from build123d import *

# Parameters (mm, degrees)
SKETCH_1_R          = 1.5
SKETCH_1_R_2        = 10
EXTRUDE_1_DEPTH     = 0.7
SKETCH_2_R          = 1.5
CUT_EXTRUDE_1_DEPTH = 40
SKETCH_4_R          = 1.5
CUT_EXTRUDE_2_DEPTH = 10


with BuildPart() as part:
    # 草图1 → 凸台-拉伸1 (new body)
    with BuildSketch(Plane.XY):
        with BuildLine():
            Line((20, 100), (-20, 100))
            ThreePointArc((-20, 100), (-76.568542495, 76.568542495), (-100, 20))
            Line((-100, 20), (-100, -80))
            ThreePointArc((-100, -80), (-94.142135624, -94.142135624), (-80, -100))
            Line((-80, -100), (80, -100))
            ThreePointArc((80, -100), (94.142135624, -94.142135624), (100, -80))
            Line((100, -80), (100, 20))
            ThreePointArc((100, 20), (76.568542495, 76.568542495), (20, 100))
        make_face()
        with Locations((-90, -90)):
            Circle(SKETCH_1_R, mode=Mode.SUBTRACT)
        with Locations((-66, -90)):
            Circle(SKETCH_1_R, mode=Mode.SUBTRACT)
        with Locations((-90, -60)):
            Circle(SKETCH_1_R, mode=Mode.SUBTRACT)
        with Locations((-66, -60)):
            Circle(SKETCH_1_R, mode=Mode.SUBTRACT)
        with Locations((-29, -90)):
            Circle(SKETCH_1_R, mode=Mode.SUBTRACT)
        with Locations((-45, -75)):
            Circle(SKETCH_1_R_2, mode=Mode.SUBTRACT)
        with Locations((-50, -36)):
            Circle(SKETCH_1_R, mode=Mode.SUBTRACT)
        with Locations((-50, -27)):
            Circle(SKETCH_1_R, mode=Mode.SUBTRACT)
        with BuildLine():
            ThreePointArc((-86.5, 35), (-85, 36.5), (-83.5, 35))
            Line((-83.5, 35), (-83.5, -35))
            ThreePointArc((-83.5, -35), (-85, -36.5), (-86.5, -35))
            Line((-86.5, -35), (-86.5, 35))
        make_face(mode=Mode.SUBTRACT)
        with Locations((-50, -18)):
            Circle(SKETCH_1_R, mode=Mode.SUBTRACT)
        with BuildLine():
            ThreePointArc((-68.5, -50), (-70, -51.5), (-71.5, -50))
            Line((-71.5, -50), (-71.5, 50))
            ThreePointArc((-71.5, 50), (-70, 51.5), (-68.5, 50))
            Line((-68.5, 50), (-68.5, -50))
        make_face(mode=Mode.SUBTRACT)
        with Locations((-50, -9)):
            Circle(SKETCH_1_R, mode=Mode.SUBTRACT)
        with Locations((-29, -41)):
            Circle(SKETCH_1_R, mode=Mode.SUBTRACT)
        with Locations((-27.275649276, -27.275649276)):
            Circle(SKETCH_1_R, mode=Mode.SUBTRACT)
        with Locations((-20.911688245, -20.911688245)):
            Circle(SKETCH_1_R, mode=Mode.SUBTRACT)
        with Locations((-14.547727215, -14.547727215)):
            Circle(SKETCH_1_R, mode=Mode.SUBTRACT)
        with Locations((-8.183766184, -8.183766184)):
            Circle(SKETCH_1_R, mode=Mode.SUBTRACT)
        with BuildLine():
            ThreePointArc((-27, -81.5), (-28.5, -80), (-27, -78.5))
            Line((-27, -78.5), (27, -78.5))
            ThreePointArc((27, -78.5), (28.5, -80), (27, -81.5))
            Line((27, -81.5), (-27, -81.5))
        make_face(mode=Mode.SUBTRACT)
        with Locations((29, -90)):
            Circle(SKETCH_1_R, mode=Mode.SUBTRACT)
        with Locations((45, -75)):
            Circle(SKETCH_1_R_2, mode=Mode.SUBTRACT)
        with BuildLine():
            Line((25, -61.5), (-25, -61.5))
            ThreePointArc((-25, -61.5), (-26.5, -60), (-25, -58.5))
            Line((-25, -58.5), (25, -58.5))
            ThreePointArc((25, -58.5), (26.5, -60), (25, -61.5))
        make_face(mode=Mode.SUBTRACT)
        with Locations((66, -90)):
            Circle(SKETCH_1_R, mode=Mode.SUBTRACT)
        with Locations((90, -90)):
            Circle(SKETCH_1_R, mode=Mode.SUBTRACT)
        with Locations((66, -60)):
            Circle(SKETCH_1_R, mode=Mode.SUBTRACT)
        with Locations((90, -60)):
            Circle(SKETCH_1_R, mode=Mode.SUBTRACT)
        with BuildLine():
            Line((50, -51.5), (-50, -51.5))
            ThreePointArc((-50, -51.5), (-51.5, -50), (-50, -48.5))
            Line((-50, -48.5), (50, -48.5))
            ThreePointArc((50, -48.5), (51.5, -50), (50, -51.5))
        make_face(mode=Mode.SUBTRACT)
        with BuildLine():
            Line((25, -41.5), (-25, -41.5))
            ThreePointArc((-25, -41.5), (-26.5, -40), (-25, -38.5))
            Line((-25, -38.5), (25, -38.5))
            ThreePointArc((25, -38.5), (26.5, -40), (25, -41.5))
        make_face(mode=Mode.SUBTRACT)
        with Locations((29, -41)):
            Circle(SKETCH_1_R, mode=Mode.SUBTRACT)
        with Locations((27.275649276, -27.275649276)):
            Circle(SKETCH_1_R, mode=Mode.SUBTRACT)
        with Locations((20.911688245, -20.911688245)):
            Circle(SKETCH_1_R, mode=Mode.SUBTRACT)
        with Locations((14.547727215, -14.547727215)):
            Circle(SKETCH_1_R, mode=Mode.SUBTRACT)
        with Locations((8.183766184, -8.183766184)):
            Circle(SKETCH_1_R, mode=Mode.SUBTRACT)
        with BuildLine():
            ThreePointArc((-50, -1.5), (-51.5, 0), (-50, 1.5))
            Line((-50, 1.5), (50, 1.5))
            ThreePointArc((50, 1.5), (51.5, 0), (50, -1.5))
            Line((50, -1.5), (-50, -1.5))
        make_face(mode=Mode.SUBTRACT)
        with Locations((50, -36)):
            Circle(SKETCH_1_R, mode=Mode.SUBTRACT)
        with Locations((50, -27)):
            Circle(SKETCH_1_R, mode=Mode.SUBTRACT)
        with Locations((50, -18)):
            Circle(SKETCH_1_R, mode=Mode.SUBTRACT)
        with Locations((50, -9)):
            Circle(SKETCH_1_R, mode=Mode.SUBTRACT)
        with Locations((-50, 9)):
            Circle(SKETCH_1_R, mode=Mode.SUBTRACT)
        with Locations((-50, 18)):
            Circle(SKETCH_1_R, mode=Mode.SUBTRACT)
        with Locations((-50, 27)):
            Circle(SKETCH_1_R, mode=Mode.SUBTRACT)
        with Locations((-50, 36)):
            Circle(SKETCH_1_R, mode=Mode.SUBTRACT)
        with Locations((-4.544155877, 4.544155877)):
            Circle(SKETCH_1_R, mode=Mode.SUBTRACT)
        with Locations((-10.908116908, 10.908116908)):
            Circle(SKETCH_1_R, mode=Mode.SUBTRACT)
        with Locations((-17.272077939, 17.272077939)):
            Circle(SKETCH_1_R, mode=Mode.SUBTRACT)
        with Locations((-23.636038969, 23.636038969)):
            Circle(SKETCH_1_R, mode=Mode.SUBTRACT)
        with Locations((-30, 30)):
            Circle(SKETCH_1_R, mode=Mode.SUBTRACT)
        with BuildLine():
            ThreePointArc((-50, 48.5), (-51.5, 50), (-50, 51.5))
            Line((-50, 51.5), (50, 51.5))
            ThreePointArc((50, 51.5), (51.5, 50), (50, 48.5))
            Line((50, 48.5), (-50, 48.5))
        make_face(mode=Mode.SUBTRACT)
        with Locations((-45, 75)):
            Circle(SKETCH_1_R_2, mode=Mode.SUBTRACT)
        with Locations((-9.77, 70.46)):
            Circle(SKETCH_1_R, mode=Mode.SUBTRACT)
        with Locations((-9.77, 90)):
            Circle(SKETCH_1_R, mode=Mode.SUBTRACT)
        with Locations((4.544155877, 4.544155877)):
            Circle(SKETCH_1_R, mode=Mode.SUBTRACT)
        with Locations((10.908116908, 10.908116908)):
            Circle(SKETCH_1_R, mode=Mode.SUBTRACT)
        with Locations((17.272077939, 17.272077939)):
            Circle(SKETCH_1_R, mode=Mode.SUBTRACT)
        with Locations((23.636038969, 23.636038969)):
            Circle(SKETCH_1_R, mode=Mode.SUBTRACT)
        with BuildLine():
            ThreePointArc((-25, 38.5), (-26.5, 40), (-25, 41.5))
            Line((-25, 41.5), (25, 41.5))
            ThreePointArc((25, 41.5), (26.5, 40), (25, 38.5))
            Line((25, 38.5), (-25, 38.5))
        make_face(mode=Mode.SUBTRACT)
        with Locations((30, 30)):
            Circle(SKETCH_1_R, mode=Mode.SUBTRACT)
        with Locations((50, 9)):
            Circle(SKETCH_1_R, mode=Mode.SUBTRACT)
        with BuildLine():
            Line((71.5, 50), (71.5, -50))
            ThreePointArc((71.5, -50), (70, -51.5), (68.5, -50))
            Line((68.5, -50), (68.5, 50))
            ThreePointArc((68.5, 50), (70, 51.5), (71.5, 50))
        make_face(mode=Mode.SUBTRACT)
        with Locations((50, 18)):
            Circle(SKETCH_1_R, mode=Mode.SUBTRACT)
        with BuildLine():
            Line((83.5, -35), (83.5, 35))
            ThreePointArc((83.5, 35), (85, 36.5), (86.5, 35))
            Line((86.5, 35), (86.5, -35))
            ThreePointArc((86.5, -35), (85, -36.5), (83.5, -35))
        make_face(mode=Mode.SUBTRACT)
        with Locations((50, 27)):
            Circle(SKETCH_1_R, mode=Mode.SUBTRACT)
        with Locations((50, 36)):
            Circle(SKETCH_1_R, mode=Mode.SUBTRACT)
        with BuildLine():
            ThreePointArc((-25, 58.5), (-26.5, 60), (-25, 61.5))
            Line((-25, 61.5), (25, 61.5))
            ThreePointArc((25, 61.5), (26.5, 60), (25, 58.5))
            Line((25, 58.5), (-25, 58.5))
        make_face(mode=Mode.SUBTRACT)
        with Locations((9.77, 70.46)):
            Circle(SKETCH_1_R, mode=Mode.SUBTRACT)
        with Locations((45, 75)):
            Circle(SKETCH_1_R_2, mode=Mode.SUBTRACT)
        with BuildLine():
            Line((27, 78.5), (-27, 78.5))
            ThreePointArc((-27, 78.5), (-28.5, 80), (-27, 81.5))
            Line((-27, 81.5), (27, 81.5))
            ThreePointArc((27, 81.5), (28.5, 80), (27, 78.5))
        make_face(mode=Mode.SUBTRACT)
        with Locations((9.77, 90)):
            Circle(SKETCH_1_R, mode=Mode.SUBTRACT)
    extrude(amount=EXTRUDE_1_DEPTH)

    # 草图2 → 切除-拉伸1 (cut)
    with BuildSketch(Plane.XY.offset(0.7)):
        with Locations((24973, 94.93)):
            Circle(SKETCH_2_R)
        with Locations((0, 89.43)):
            Circle(SKETCH_2_R)
        with Locations((12.929759279, 67.035)):
            Circle(SKETCH_2_R)
        with Locations((-12.929759279, 67.035)):
            Circle(SKETCH_2_R)
        with Locations((0, 74.5)):
            Circle(SKETCH_2_R)
    extrude(amount=-CUT_EXTRUDE_1_DEPTH, mode=Mode.SUBTRACT)

    # 草图4 → 切除-拉伸2 (cut)
    with BuildSketch(Plane.XY.offset(0.7)):
        with Locations((0, 96)):
            Circle(SKETCH_4_R)
        with Locations((-30.608507012, 90)):
            Circle(SKETCH_4_R)
        with Locations((30.608507012, 90)):
            Circle(SKETCH_4_R)
    extrude(amount=-CUT_EXTRUDE_2_DEPTH, mode=Mode.SUBTRACT)


solid = part.part
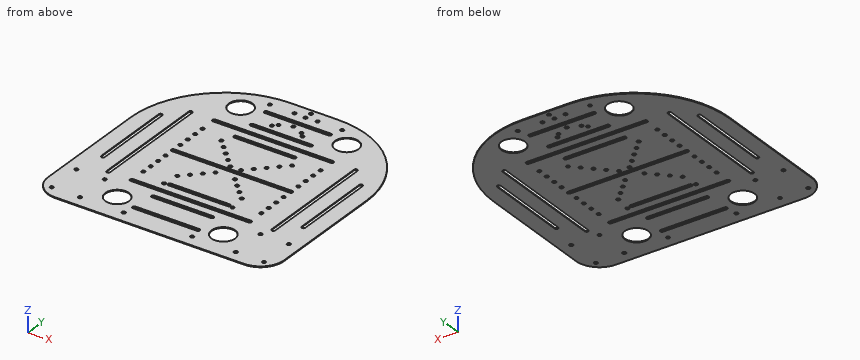
The model under review builds one solid part; all positions refer to its coordinate system, in mm. Round coordinates to 2 decimals unless told otherwise and drop trailing zeros. Loops run counter-clockwise (first coordinate to the right, second up) from the corner with the lowest first, then second, coordinate; pieces in that order, holes last. Notation, with made-up numbers: (3.25, 29) -> (53.25, 29) arc R17 cw to (53.25, 61) -> close; hole circle Ø8 at (11.5, 12). An arc over 180 degrees is marked (long way). Write item = value, one per line. Start each with the question number.
Item 1: Take a section at D-D on x = 60. Give the boundary of the cut face in (y, z).
Item 2: Take a section at C-C on z = 0.3. Count the separate pieces of the cut face and the enclosed holes in it, plus the area to 3 significant figures.
Item 3: Insertion check: pin 1 (2.5 mm diameter, centred on x = 14.55, y = -14.55, fed in from +Z). The pin has a flat end and moves straight along its axis. Give the tip position at first contact, or say it passes through.
Item 4: To check wall thickness, follow L1, parallel to X at y = -43.5, z = 0.2; L2, parallel to X at y = 81, z = 0.55; L3, parallel to X at y = 45, z = 0.25. State the ranges of each line that lie inside material, in increasing order.
Item 5: Take a section at A-A on x = -45. Give the boundary of the cut face in (y, z), plus the area to 3 significant figures.
Item 6: Take a section at B-B on x = 40. Give the boundary of the cut face in (y, z), plus the area to 3 significant figures.
Result:
q1.outline = (-100, 0) -> (89.28, 0) -> (89.28, 0.7) -> (-100, 0.7) -> close
q2.separate_pieces = 1
q2.enclosed_holes = 74
q2.area = 32,500 mm²
q3.pin_1 = through
q4.L1 = -100 to -71.5, -68.5 to 68.5, 71.5 to 100
q4.L2 = -71.76 to -53, -37 to -28.12, 28.12 to 37, 53 to 71.76
q4.L3 = -95.99 to -71.5, -68.5 to 68.5, 71.5 to 95.99
q5.outline = (-100, 0) -> (-85, 0) -> (-85, 0.7) -> (-100, 0.7) -> close; (-65, 0) -> (-51.5, 0) -> (-51.5, 0.7) -> (-65, 0.7) -> close; (-48.5, 0) -> (-1.5, 0) -> (-1.5, 0.7) -> (-48.5, 0.7) -> close; (1.5, 0) -> (48.5, 0) -> (48.5, 0.7) -> (1.5, 0.7) -> close; (51.5, 0) -> (65, 0) -> (65, 0.7) -> (51.5, 0.7) -> close; (85, 0) -> (95.99, 0) -> (95.99, 0.7) -> (85, 0.7) -> close
q5.area = 103 mm²
q6.outline = (-100, 0) -> (-83.66, 0) -> (-83.66, 0.7) -> (-100, 0.7) -> close; (-66.34, 0) -> (-51.5, 0) -> (-51.5, 0.7) -> (-66.34, 0.7) -> close; (-48.5, 0) -> (-1.5, 0) -> (-1.5, 0.7) -> (-48.5, 0.7) -> close; (1.5, 0) -> (48.5, 0) -> (48.5, 0.7) -> (1.5, 0.7) -> close; (51.5, 0) -> (66.34, 0) -> (66.34, 0.7) -> (51.5, 0.7) -> close; (83.66, 0) -> (97.46, 0) -> (97.46, 0.7) -> (83.66, 0.7) -> close
q6.area = 108 mm²
